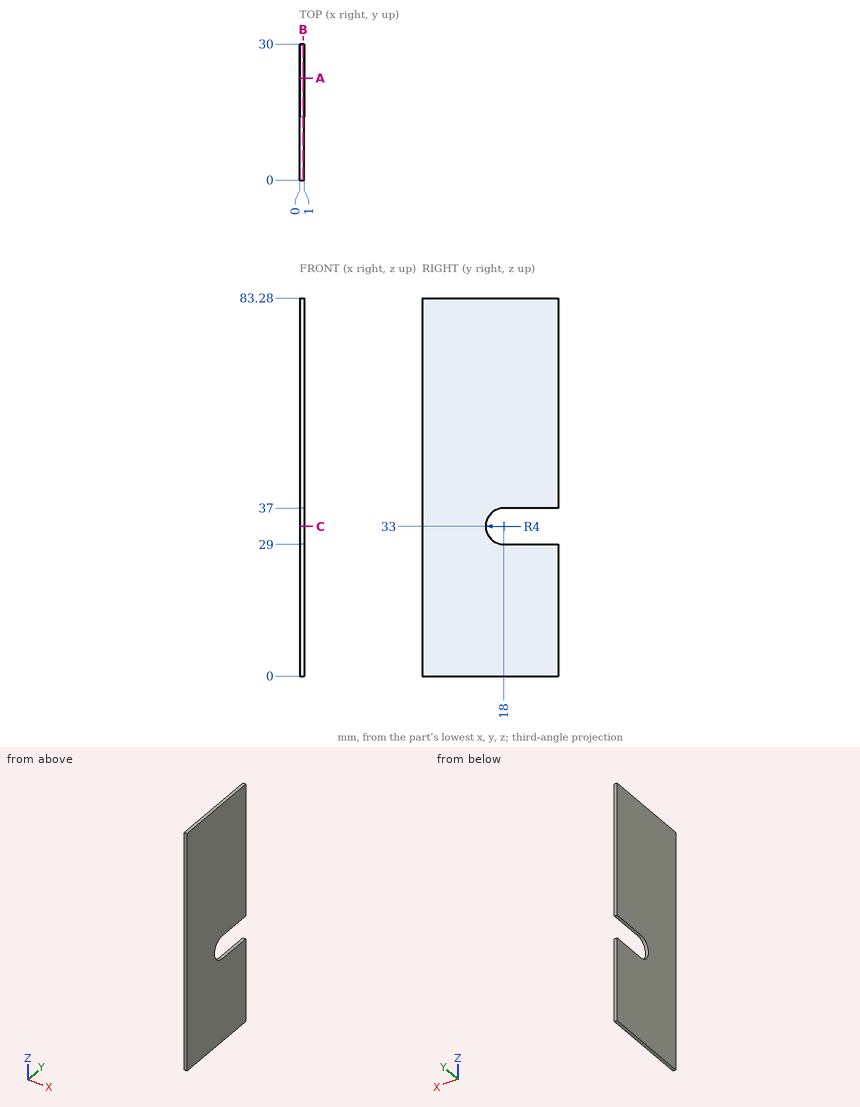
Check sheet for the drawn part. Datum: minimum x, y, z corner. Units: mm. Coordinates: 2 decimals unless noted, no trailing zeros. Order: outer loops, then holes, each group sorted by start corner. A loop starts at its lowest first (then second) coordinate and runs counter-clockwise, first axis right, second up. Notation, with made-up numbers: M 29,66 L 76,66 A9 cw 76,83 Z; hole C 35.25,32.25 d6. An arc over 180 degrees is marked long. One line per question, with ' | ' between items. Start each with the question number.
Item 1: Material ranges on L1, parallel to Z at x = 0.95, y = 21.25; L2, parallel to Y at x = 0.2, z = 33.5, recorded low to high. Write a range as [from, to].
Item 2: Cross-section at B-B on x = 0.75. Enter the section's corners in (y, z), then the cut area to 3 significant figures.
Item 3: Cross-section at A-A on y = 22.5. Enter the section's corners in (x, z), then the cut area to 3 significant figures.
Item 4: Cross-section at C-C on z = 33. Enter the section's corners in (x, y), then the cut area to 3 significant figures.
Findings:
1) L1: z = [0, 29], [37, 83.28] | L2: y = [0, 14.03]
2) outline: M 0,0 L 30,0 L 30,29 L 18,29 A4 cw 18,37 L 30,37 L 30,83.28 L 0,83.28 Z | area: 2,380 mm²
3) outline: M 0,0 L 1,0 L 1,29 L 0,29 Z; M 0,37 L 1,37 L 1,83.28 L 0,83.28 Z | area: 75.3 mm²
4) outline: M 0,0 L 1,0 L 1,14 L 0,14 Z | area: 14.0 mm²
